Part model, mm, in its own coordinate system. A direction names the side the tool comes from. Give positions to 0.01 mm unless a question says otherwise; leave off trailing zeros. Order: outer loops, then holes, each group sorted by start corner. A loop starts at its lowest first (then second) coordinate and runs counter-clockwise, first axis right, second up. Notation, with made-up numbers: M 72,81.5 L 130,81.5 A33 cw 130,117.5 Z; hole C -33,73.25 d1. An arc over 180 degrees is marked long. Answer as a JSON object with one key per item and string values.
from build123d import *

# Parameters (mm, degrees)
SKETCH_1_W               = 71.4
SKETCH_1_H               = 59
EXTRUDE_1_DEPTH          = 3.5
CUT_EXTRUDE_4_DEPTH      = 8.5
CUT_EXTRUDE_4_DEPTH_BACK = 15
SKETCH_2_R               = 1.45
SKETCH_5_W               = 26.11
SKETCH_5_H               = 45.8
EXTRUDE_2_DEPTH          = 10.15
SKETCH_6_W               = 20
SKETCH_6_H               = 39.55
CUT_EXTRUDE_5_DEPTH      = 10.15


with BuildPart() as part:
    # 草圖1 → 填料-伸長1 (new body)
    with BuildSketch(Plane(origin=(0, 0, 0), x_dir=(1, 0, 0), z_dir=(0, 1, 0))):
        Rectangle(SKETCH_1_W, SKETCH_1_H)
    extrude(amount=-EXTRUDE_1_DEPTH)

    # 草圖2 → 除料-伸長4 (cut, two sides: drawn at the far end of the back side and taken through both)
    with BuildSketch(Plane(origin=(0, 0, 0), x_dir=(1, 0, 0), z_dir=(0, 1, 0)).offset(-CUT_EXTRUDE_4_DEPTH_BACK)):
        with Locations(Location((20.453418067, -24.130543915, 0), (0, 0, 270))):
            Circle(SKETCH_2_R)
        with Locations(Location((-30.223577589, 18.9, 0), (0, 0, 270))):
            Circle(SKETCH_2_R)
        with Locations(Location((-30.223577589, -8.577967438, 0), (0, 0, 270))):
            Circle(SKETCH_2_R)
        with Locations(Location((21.85, 24.05, 0), (0, 0, 270))):
            Circle(SKETCH_2_R)
    extrude(amount=CUT_EXTRUDE_4_DEPTH + CUT_EXTRUDE_4_DEPTH_BACK, mode=Mode.SUBTRACT)

    # 草圖5 → 填料-伸長2 (add)
    with BuildSketch(Plane(origin=(0, -3.5, 0), x_dir=(-1, 0, 0), z_dir=(0, -1, 0))):
        Rectangle(SKETCH_5_W, SKETCH_5_H)
    extrude(amount=EXTRUDE_2_DEPTH)

    # 草圖6 → 除料-伸長5 (cut)
    with BuildSketch(Plane.XZ.offset(13.65)):
        Rectangle(SKETCH_6_W, SKETCH_6_H)
    extrude(amount=-CUT_EXTRUDE_5_DEPTH, mode=Mode.SUBTRACT)


solid = part.part
1. Probe line 1 along X through (y, z) = (-1.9, -18.9); line 2 along X through (y, z) = (-9.5, -2) (3 decimals); line 3 along Z through (x, y) = (1, -11.25) (3 decimals). List the from-to ranges inside material, lowest first.
Worked answers:
{"line 1": "x = -35.7 to -31.67, -28.77 to 35.7", "line 2": "x = -13.055 to -10, 10 to 13.055", "line 3": "z = -22.9 to -19.775, 19.775 to 22.9"}
2. Cut at B-B on x = 8.5. Give the cut face in (y, z) (3 decimals).
Worked answers:
{"outline": "M -13.65,-22.9 L -3.5,-22.9 L -3.5,-29.5 L 0,-29.5 L 0,29.5 L -3.5,29.5 L -3.5,22.9 L -13.65,22.9 L -13.65,19.775 L -3.5,19.775 L -3.5,-19.775 L -13.65,-19.775 Z"}
3. Cut at C-C on y = -5. Give the cut face in (x, z) (3 decimals).
Worked answers:
{"outline": "M -13.055,-22.9 L 13.055,-22.9 L 13.055,22.9 L -13.055,22.9 Z; hole M -10,-19.775 L 10,-19.775 L 10,19.775 L -10,19.775 Z"}
4. Pin check, flat tips, straight feed: P1, Ø2.5, axis at x = -30.22, z = 8.58, coming from the -Y side; P2, Ø3, axis at y = -6, z = -0.5, coming from the +X side (3 decimals); P3, Ø10, axis at x = -3, z = -6, coming from the -Y side; P4, Ø8, axis at y = -9.5, z = 0.5, coming from the -X side (3 decimals). Stop position of each tip, or through.
Worked answers:
{"P1": "passes through", "P2": "stops at x = 13.055", "P3": "stops at y = -3.5", "P4": "stops at x = -13.055"}
5. Cut at A-A on z = -24.05. Give the cut face in (x, y).
Worked answers:
{"outline": "M -35.7,-3.5 L 20.4,-3.5 L 20.4,0 L -35.7,0 Z; M 23.3,-3.5 L 35.7,-3.5 L 35.7,0 L 23.3,0 Z"}
6. Cut at D-D on z = -14.5. Give the cut face in (x, y) (3 decimals), plus the area to 3 significant figures.
Worked answers:
{"outline": "M -35.7,-3.5 L -13.055,-3.5 L -13.055,-13.65 L -10,-13.65 L -10,-3.5 L 10,-3.5 L 10,-13.65 L 13.055,-13.65 L 13.055,-3.5 L 35.7,-3.5 L 35.7,0 L -35.7,0 Z", "area": "312 mm^2"}
7. Which spindle directions (+Z, -Z, +X, -X, +Y, -Y) get a long thin tool onto all of the face, cutting with end or side? Do faces 1 (the flat face through (0, -9, -22.9)), 2 (the flat face through (0, -9, 19.775)), 3 (the flat face through (-13.055, -9, 0)). Say none if no direction does.
Worked answers:
{"face 1": "-Z, +X, -X, -Y", "face 2": "-Y", "face 3": "+Z, -Z, -X, -Y"}
